```python
from build123d import *

# Parameters (mm, degrees)
F0_R     = 12.7
F0_R_2   = 11.1125
F1_DEPTH = 254
F3_DEPTH = 25.4


with BuildPart() as f1:
    # F0 (on Top) → F1 (new body, symmetric)
    with BuildSketch(Plane.XY):
        Circle(F0_R)
        Circle(F0_R_2, mode=Mode.SUBTRACT)
    extrude(amount=F1_DEPTH, both=True)

    # F2 (on Front) → F3 (cut)
    with BuildSketch(Plane.XZ):
        with BuildLine():
            Line((4.699, 190.5), (-4.699, 190.5))
            ThreePointArc((-4.699, 190.5), (-5.866433, 190.016433), (-6.35, 188.849))
            Line((-6.35, 188.849), (-6.35, 166.751))
            ThreePointArc((-6.35, 166.751), (-5.866433, 165.583567), (-4.699, 165.1))
            Line((-4.699, 165.1), (4.699, 165.1))
            ThreePointArc((4.699, 165.1), (5.866433, 165.583567), (6.35, 166.751))
            Line((6.35, 166.751), (6.35, 188.849))
            ThreePointArc((6.35, 188.849), (5.866433, 190.016433), (4.699, 190.5))
        make_face()
    extrude(amount=F3_DEPTH, mode=Mode.SUBTRACT)


solid = f1.part
```
Here's how the part is built. I have some questions about the finished solid (model axes, mm). Round coordinates to 2 decimals unless told otherwise and drop trailing zeros. Order: outer loops, then holes, each group sorted by start corner. A loop starts at its lowest first (then second) coordinate and runs counter-clockwise, first axis right, second up. Notation, with made-up numbers: (-7.75, 70.5) -> (35.25, 70.5) arc R20 ccw to (35.25, 77.5) -> close; hole circle Ø9 at (57.5, 51.5). An arc over 180 degrees is marked (long way). Use a Markdown table: item, result. Add a question column.
(1) If we mould it in two halves opening along Y, with no side actions, what happens to faces 1 (the face through (-1.447, 11.018, -3.556)), 2 (the face through (-1.653, 12.592, 3.556)), 3 (the face through (0.88, -11.23, 254))? For each: released by +Y, released by -Y, zero draft, split by the parting line, or undercut.
(2) Suppose I cut it at C-C, the plane z = -14.5. Please give me the cut outline in (x, y) (1 decimal), and give its area (3 significant figures).
(3) For pin 1 Ø0.9 at (y, z) = (-9.5, 174) entering from +X; pin 2 Ø3 at (x, y) = (1, -11) entering from -Z; pin 3 Ø0.6 at (y, z) = (-10, 178.5) entering from -X; pin 4 Ø4 at (x, z) = (9.5, -148) entering from -Y, each with a flat end and sliding along its axis, tell me the tip position at first contact or that it passes through.
(4) Suppose I cut it at B-B, the plane x = 0. Please give me the cut outline in (y, z).
(5) I need wall thicknesses on line 1 along Y through (x, z) = (0, -38.5); line 2 along X through (y, z) = (-6.5, 47); line 3 along Y through (x, z) = (-8.75, -121.5). Which ranges of each line are inside material? Lowest first, please.
(6) Suppose I cut it at A-A, the plane y = 0. Please give me the cut outline in (x, z).
Verdict:
| question | item | result |
|---|---|---|
| 1 | face 1 | undercut |
| 1 | face 2 | split by the parting line |
| 1 | face 3 | zero draft |
| 2 | outline | circle Ø25.4 at (0, 0); hole circle Ø22.2 at (0, 0) |
| 2 | area | 119 mm2 |
| 3 | pin 1 | x = 8.91 |
| 3 | pin 2 | z = -254 |
| 3 | pin 3 | x = -8.2 |
| 3 | pin 4 | y = -10.25 |
| 4 | outline | (-12.7, -254) -> (-11.11, -254) -> (-11.11, 165.1) -> (-12.7, 165.1) -> close; (-12.7, 190.5) -> (-11.11, 190.5) -> (-11.11, 254) -> (-12.7, 254) -> close; (11.11, -254) -> (12.7, -254) -> (12.7, 254) -> (11.11, 254) -> close |
| 5 | line 1 | -12.7 to -11.11, 11.11 to 12.7 |
| 5 | line 2 | -10.91 to -9.01, 9.01 to 10.91 |
| 5 | line 3 | -9.2 to -6.85, 6.85 to 9.2 |
| 6 | outline | (-12.7, -254) -> (-11.11, -254) -> (-11.11, 254) -> (-12.7, 254) -> close; (11.11, -254) -> (12.7, -254) -> (12.7, 254) -> (11.11, 254) -> close |
